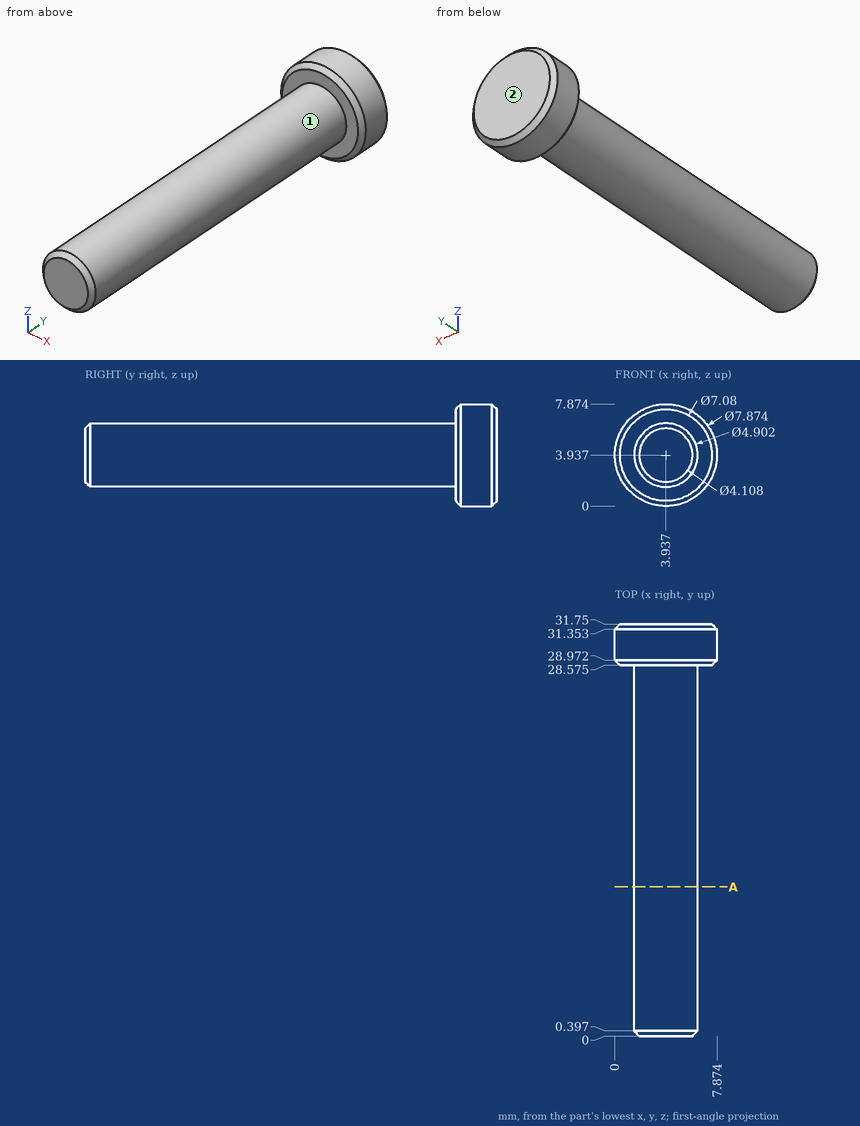
Geometry: see drawing. Coordinates: mm, zero at the bounding-box minimum. A direction names the side the tool comes from. Round coordinates to 2 decimals unless told otherwise and drop trailing zeros. Loops run counter-clockwise (first coordinate to the right, second up) from the corner with the lowest first, then second, coordinate; pieces in that order, holes last. Notation, with made-up numbers: (-17.75, 28.25) -> (21.25, 28.25) arc R15 ccw to (21.25, 53.25) -> close; hole circle Ø6 at (-12.75, 85). An arc over 180 degrees is marked (long way). Write each question's results on one line, items separated by ' | '.
1. Section A-A (y = 11.5). Return loops of the section in (x, z) (1 decimal), and give its area (3 significant figures).
Geometry results:
outline: circle Ø4.9 at (3.9, 3.9) | area: 18.9 mm2
2. Set-up query: the marked faces 1 and 2. Return all of +Z, -Z, +X, -X, +Y, -Y with unobstructed straight access to the full face (end or side cutting, diameter ignored); none if empty.
Geometry results:
face 1: -Y | face 2: +Z, -Z, +X, -X, +Y
3. First-contact query: P1, Ø1, axis at y = 3.5, z = 5.5, coming from the +X side (1 decimal); P2, Ø2, axis at y = 17, z = 1, coming from the +X side; P3, Ø4, axis at y = 22, z = 5, coming from the -X side. Flat tips, straight axial feed; report the tip coordinate or a pass-through.
Geometry results:
P1: x = 6.1 | P2: x = 5.44 | P3: x = 1.49
4. Ray query, line 1 (X direction, y = 8.5, z = 3.75); line 2 (Z direction, x = 2.5, y = 13); line 3 (Y direction, x = 6, z = 7) (1 decimal). Return the intervals inside material, ascending. Write a range as from..to.
Geometry results:
line 1: 1.49..6.38 | line 2: 1.95..5.92 | line 3: 28.7..31.6
